```python
from build123d import *

# Parameters (mm, degrees)
CROQUIS2_R              = 30
SALIENTE_EXTRUIR1_DEPTH = 5
CROQUIS6_R              = 23.5
SALIENTE_EXTRUIR5_DEPTH = 5.5
CROQUIS7_W              = 3
CROQUIS7_H              = 34
SALIENTE_EXTRUIR6_DEPTH = 23.4
REDONDEO1_R             = 3
CROQUIS8_R              = 10.15
CORTAR_EXTRUIR1_DEPTH   = 5
CORTAR_EXTRUIR2_REACH   = 53.054
CROQUIS9_R              = 1.25
CROQUIS10_R             = 1.5
CORTAR_EXTRUIR3_DEPTH   = 3.5
CORTAR_EXTRUIR4_REACH   = 50.452
CROQUIS11_R             = 4.998325146
CORTAR_EXTRUIR5_REACH   = 61.737
CROQUIS12_W             = 5
CROQUIS12_H             = 9.9
CROQUIS13_W             = 26.3
CROQUIS13_H             = 4.3
SALIENTE_EXTRUIR7_DEPTH = 2.3
REDONDEO2_R             = 2.3
CORTAR_EXTRUIR6_DEPTH   = 2.3
CROQUIS16_R             = 1
CORTAR_EXTRUIR7_DEPTH   = 2.3
CROQUIS17_R             = 1.65
CORTAR_EXTRUIR8_DEPTH   = 1


with BuildPart() as part:
    # Croquis2 → Saliente-Extruir1 (new body)
    with BuildSketch(Plane.XY):
        Circle(CROQUIS2_R)
    extrude(amount=SALIENTE_EXTRUIR1_DEPTH)

    # Croquis6 → Saliente-Extruir5 (add)
    with BuildSketch(Plane(origin=(0, 0, 0), x_dir=(-1, 0, 0), z_dir=(0, 0, -1))):
        Circle(CROQUIS6_R)
    extrude(amount=SALIENTE_EXTRUIR5_DEPTH)

    # Croquis7 → Saliente-Extruir6 (add)
    with BuildSketch(Plane.XY.offset(5)):
        with Locations((-11.65, -7.5)):
            Rectangle(CROQUIS7_W, CROQUIS7_H)
        with Locations((11.65, -7.5)):
            Rectangle(CROQUIS7_W, CROQUIS7_H)
    extrude(amount=SALIENTE_EXTRUIR6_DEPTH)

    # Redondeo1
    redondeo1_edges = [part.edges().sort_by_distance(p)[0] for p in [
        (13.15, -24.5, 16.7),
        (-13.15, -24.5, 16.7),
    ]]
    fillet(redondeo1_edges, radius=REDONDEO1_R - 0.0001)  # a hair under: the kernel refuses the full size

    # Croquis8 → Cortar-Extruir1 (cut)
    with BuildSketch(Plane.XY.offset(5)):
        Circle(CROQUIS8_R)
    extrude(amount=-CORTAR_EXTRUIR1_DEPTH, mode=Mode.SUBTRACT)

    # Croquis9 → Cortar-Extruir2 (cut, up to next)
    with BuildSketch(Plane.XY, mode=Mode.PRIVATE) as cortar_extruir2_sk1:
        with Locations((0, 5.5)):
            Circle(CROQUIS9_R)
    cortar_extruir2_tool1 = extrude(cortar_extruir2_sk1.sketch, amount=-CORTAR_EXTRUIR2_REACH, mode=Mode.PRIVATE) & part.part
    # Croquis9 → Cortar-Extruir2 (cut, up to next)
    with BuildSketch(Plane.XY, mode=Mode.PRIVATE) as cortar_extruir2_sk2:
        with Locations((5.5, 0)):
            Circle(CROQUIS9_R)
    cortar_extruir2_tool2 = extrude(cortar_extruir2_sk2.sketch, amount=-CORTAR_EXTRUIR2_REACH, mode=Mode.PRIVATE) & part.part
    # Croquis9 → Cortar-Extruir2 (cut, up to next)
    with BuildSketch(Plane.XY, mode=Mode.PRIVATE) as cortar_extruir2_sk3:
        with Locations((0, -5.5)):
            Circle(CROQUIS9_R)
    cortar_extruir2_tool3 = extrude(cortar_extruir2_sk3.sketch, amount=-CORTAR_EXTRUIR2_REACH, mode=Mode.PRIVATE) & part.part
    # Croquis9 → Cortar-Extruir2 (cut, up to next)
    with BuildSketch(Plane.XY, mode=Mode.PRIVATE) as cortar_extruir2_sk4:
        with Locations((-5.5, 0)):
            Circle(CROQUIS9_R)
    cortar_extruir2_tool4 = extrude(cortar_extruir2_sk4.sketch, amount=-CORTAR_EXTRUIR2_REACH, mode=Mode.PRIVATE) & part.part
    add(cortar_extruir2_tool1.solids().sort_by_distance((0, 5.5, 0))[0], mode=Mode.SUBTRACT)
    add(cortar_extruir2_tool2.solids().sort_by_distance((5.5, 0, 0))[0], mode=Mode.SUBTRACT)
    add(cortar_extruir2_tool3.solids().sort_by_distance((0, -5.5, 0))[0], mode=Mode.SUBTRACT)
    add(cortar_extruir2_tool4.solids().sort_by_distance((-5.5, 0, 0))[0], mode=Mode.SUBTRACT)

    # Croquis10 → Cortar-Extruir3 (cut)
    with BuildSketch(Plane.XY.offset(5)):
        with Locations((21.650635095, -12.5)):
            Circle(CROQUIS10_R)
        with Locations((-21.650635095, -12.5)):
            Circle(CROQUIS10_R)
        with Locations((21.650635095, 12.5)):
            Circle(CROQUIS10_R)
        with Locations((-21.650635095, 12.5)):
            Circle(CROQUIS10_R)
        with Locations((0, 25)):
            Circle(CROQUIS10_R)
    extrude(amount=-CORTAR_EXTRUIR3_DEPTH, mode=Mode.SUBTRACT)

    # Croquis11 → Cortar-Extruir4 (cut, up to next)
    with BuildSketch(Plane.XY.offset(5), mode=Mode.PRIVATE) as cortar_extruir4_sk1:
        with Locations(Location((0, 12, 0), (0, 0, 326.642787388))):
            Circle(CROQUIS11_R)
    cortar_extruir4_tool1 = extrude(cortar_extruir4_sk1.sketch, amount=-CORTAR_EXTRUIR4_REACH, mode=Mode.PRIVATE) & part.part
    add(cortar_extruir4_tool1.solids().sort_by_distance((0, 12, 5))[0], mode=Mode.SUBTRACT)

    # Cortar-Extruir5: up to this face of the body (flat: up to its plane)
    cortar_extruir5_end = Plane(part.part.faces().sort_by_distance((-13.15, -6.00005, 16.7))[0])
    # Croquis12 → Cortar-Extruir5 (cut, up to the picked face)
    with BuildSketch(Plane(origin=(13.15, 0, 0), x_dir=(0, 0, -1), z_dir=(1, 0, 0)), mode=Mode.PRIVATE) as cortar_extruir5_sk1:
        with Locations((-7.5, -9)):
            Rectangle(CROQUIS12_W, CROQUIS12_H)
    cortar_extruir5_tool1 = split(extrude(cortar_extruir5_sk1.sketch, amount=-CORTAR_EXTRUIR5_REACH, mode=Mode.PRIVATE), bisect_by=cortar_extruir5_end, keep=Keep.BOTH, mode=Mode.PRIVATE)
    add(cortar_extruir5_tool1.solids().sort_by(Axis((13.15, -9, 7.5), (-1, 0, 0)))[0], mode=Mode.SUBTRACT)

    # Croquis13 → Saliente-Extruir7 (add)
    with BuildSketch(Plane.XY.offset(28.4)):
        with Locations((0, 7.35)):
            Rectangle(CROQUIS13_W, CROQUIS13_H)
    extrude(amount=SALIENTE_EXTRUIR7_DEPTH)

    # Redondeo2
    redondeo2_edges = [part.edges().sort_by_distance(p)[0] for p in [
        (11.65, 5.2, 28.4),
        (-11.65, 5.2, 28.4),
    ]]
    fillet(redondeo2_edges, radius=REDONDEO2_R - 0.0001)  # a hair under: the kernel refuses the full size

    # Croquis15 → Cortar-Extruir6 (cut)
    with BuildSketch(Plane.XY.offset(30.7)):
        with BuildLine():
            Line((-7.082372484, 4.7), (7.082372484, 4.7))
            ThreePointArc((7.082372484, 4.7), (0, 8.5), (-7.082372484, 4.7))
        make_face()
    extrude(amount=-CORTAR_EXTRUIR6_DEPTH, mode=Mode.SUBTRACT)

    # Croquis16 → Cortar-Extruir7 (cut)
    with BuildSketch(Plane.XY.offset(30.7)):
        with Locations((-8, 7.5)):
            Circle(CROQUIS16_R)
        with Locations((8, 7.5)):
            Circle(CROQUIS16_R)
    extrude(amount=-CORTAR_EXTRUIR7_DEPTH, mode=Mode.SUBTRACT)

    # Croquis17 → Cortar-Extruir8 (cut)
    with BuildSketch(Plane.XY.offset(30.7)):
        with Locations((-8, 7.5)):
            Circle(CROQUIS17_R)
        with Locations((8, 7.5)):
            Circle(CROQUIS17_R)
    extrude(amount=-CORTAR_EXTRUIR8_DEPTH, mode=Mode.SUBTRACT)


solid = part.part
```
Verification items for the finished model (mm, model axes). A direction names the side the tool comes from. Coordinates: 2 decimals unless noted, no trailing zeros. Order: outer loops, then holes, each group sorted by start corner. A loop starts at its lowest first (then second) coordinate and runs counter-clockwise, first axis right, second up. Notation, with made-up numbers: (40, 8.25) -> (85, 8.25) arc R24 ccw to (85, 33.25) -> close; hole circle Ø4 at (64.5, 67.5). An arc over 180 degrees is marked (long way). Answer as CSV lines item,"result". Start each with the question number.
1) Cross-section at B-B, the plane x = 0. Give the number of separate pieces and of enclosed holes in the cut face, then the cut area to 3 significant figures.
2) Material ranges on L1, parallel to Y at x = 0, z = 3.55; L2, parallel to Y at x = 8, z = 29.1; L3, parallel to Y at x = 0, z = 1, recorded low to high. Write a range as [from, to].
3) Release check for a two-part mould opening along X. For faces 4 (the face through (-8.13, 8.49, 29.06)), 5 (the face through (-13.15, -6, 18)), 6 (the face through (-8, 6, 29.7)), 7 (the face through (12, -11, 28.4)) record: released by +X, released by -X, zero draft, split by the parting line, or undercut.
4) Set-up check for faces 1 (the face through (23.08, -12.05, 3.27)), 2 (the face through (13, -20, 0)), 3 (the face through (-0.386, -10.143, 2.535)): record each of +Z, -Z, +X, -X, +Y, -Y from which the full face is reachable in a straight line by a thin tool's end or side.
5) Cross-section at D-D, the plane x = 8. Record the boundary of the cut face in (y, z).
6) Gauge pin test, flat ends, axial feed: pin 1 Ø1.5 at (y, z) = (-6, 2.5) entering from -X; pin 2 Ø4 at (x, y) = (-15, -13.5) entering from +Z; pin 3 Ø3 at (x, y) = (-8, 7.5) entering from +Z. Record the tip position at first contact, or that the pin passes through.
Conclusion:
1,separate pieces,"5"
1,enclosed holes,"0"
1,area,"332 mm²"
2,L1,"y = [-30, -10.15], [17, 23.5], [26.5, 30]"
2,L2,"y = [5.2, 6.5], [8.5, 9.5]"
2,L3,"y = [-30, -10.15], [17, 30]"
3,face 4,"undercut"
3,face 5,"released by -X"
3,face 6,"undercut"
3,face 7,"zero draft"
4,face 1,"+Z"
4,face 2,"-Z"
4,face 3,"none"
5,outline,"(-28.91, 0) -> (-22.1, 0) -> (-22.1, -5.5) -> (22.1, -5.5) -> (22.1, 0) -> (28.91, 0) -> (28.91, 5) -> (6.25, 5) -> (6.25, 0) -> (-6.25, 0) -> (-6.25, 5) -> (-28.91, 5) -> close; (5.2, 28.4) -> (6.5, 28.4) -> (6.5, 29.7) -> (5.85, 29.7) -> (5.85, 30.7) -> (5.2, 30.7) -> close; (8.5, 28.4) -> (9.5, 28.4) -> (9.5, 30.7) -> (9.15, 30.7) -> (9.15, 29.7) -> (8.5, 29.7) -> close"
6,pin 1,"stops at x = -29.54"
6,pin 2,"stops at z = 28.4"
6,pin 3,"stops at z = 29.7"
